Geometry check sheet. Reference: drawing and pictorial views, mm from the part's lowest x, y, z. Round coordinates to 2 decimals unless told otherwise and drop trailing zeros. Order: outer loops, then holes, each group sorted by start corner. A loop starts at its lowest first (then second) coordinate and runs counter-clockwise, first axis right, second up.
(1) Thickness scan on probe 1 along Y at (x, z) = (12.5, 13.75); probe 2 along X at (y, z) = (13.25, 3); probe 3 along X at (y, z) = (2.5, 13.5). Record the ranges inside material, lowest first.
(2) Sectioned sample at A-A, the plane z = 17.25. Enter the section's corners in (x, y), and give its area (3 significant figures).
(3) Sectioned sample at B-B, the plane y = 6. Enter the section's corners in (x, z).
(4) Sectioned sample at C-C, the plane y = 20.25. Enter the section's corners in (x, z).
(5) Depth check by flat-ended pin: pin 1 (6 mm diameter, centred on y = 17, z = 17, fed in from +X); pin 2 (10 mm diameter, centred on y = 22, z = 16.5, fed in from -X). Enter the tip coordinate at first touch or a pass-through.
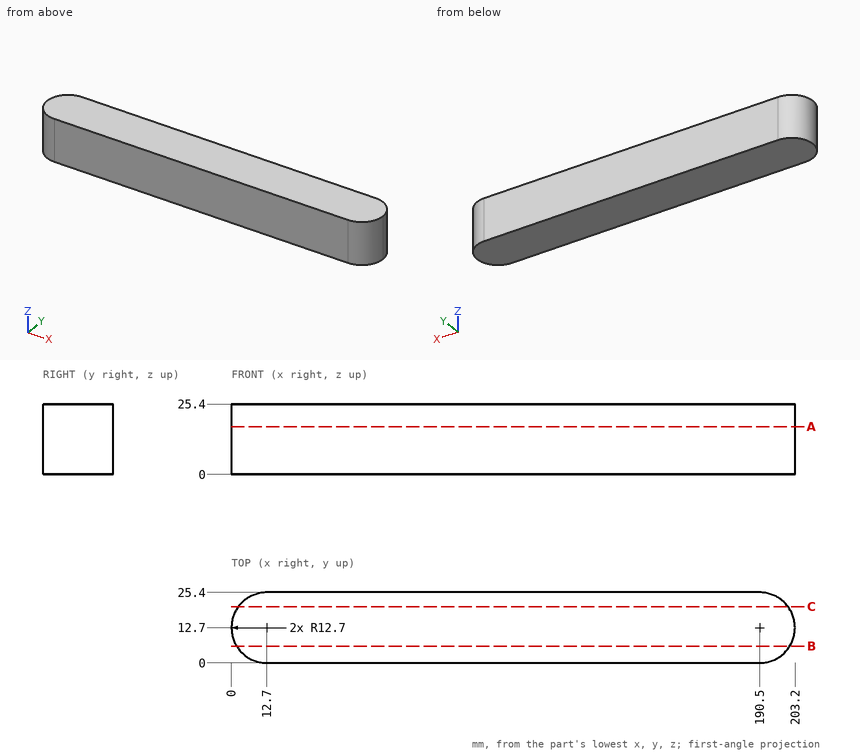
Derived:
1. probe 1: y = 0 to 25.4
1. probe 2: x = 0.01 to 203.19
1. probe 3: x = 5.13 to 198.07
2. outline: (12.7, 0) - (190.5, 0) arc R12.7 ccw to (190.5, 25.4) - (12.7, 25.4) arc R12.7 ccw to start
2. area: 5,020 mm2
3. outline: (1.91, 0) - (201.29, 0) - (201.29, 25.4) - (1.91, 25.4) - close
4. outline: (2.49, 0) - (200.71, 0) - (200.71, 25.4) - (2.49, 25.4) - close
5. pin 1: stops at x = 203.13
5. pin 2: stops at x = 0.75
